from build123d import *

# Parameters (mm, degrees)
F1_DEPTH = 5
F3_D     = 5


with BuildPart() as f1:
    # F0 (on Top) → F1 (new body)
    with BuildSketch(Plane.XY):
        with BuildLine():
            Line((-14.706516, -4.991379), (-0.002931, -4.999999))
            ThreePointArc((-0.002931, -4.999999), (3.536527, -3.53454), (4.999997, 0.005741))
            Line((4.999997, 0.005741), (4.98325, 14.591081))
            Line((4.98325, 14.591081), (4.982298, 15.420361))
            ThreePointArc((4.982298, 15.420361), (-0.210367, 19.995573), (-5, 15))
            ThreePointArc((-5, 15), (-7.928932, 7.928932), (-15, 5))
            ThreePointArc((-15, 5), (-19.997844, -0.146805), (-14.706516, -4.991379))
        make_face()
        with BuildLine():
            Line((4.982298, 15.420361), (4.98325, 14.591081))
            ThreePointArc((4.98325, 14.591081), (4.999997, 15.005741), (4.982298, 15.420361))
        make_face()
    extrude(amount=F1_DEPTH)

    # F3 (through all)
    with Locations(Plane.XY.offset(5)):
        with Locations((0, 15), (-15, 0)):
            Hole(F3_D / 2)


solid = f1.part
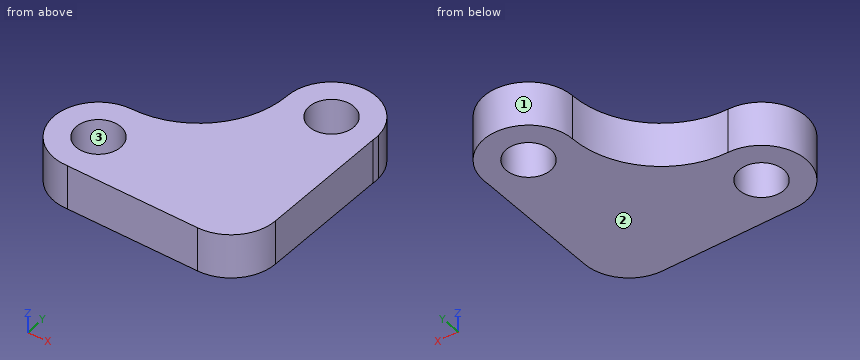
Model file for the job. Use its own axes, mm. Face numbers are marked on the shaded views. Give positions to 0.01 mm unless a question says otherwise; leave off trailing zeros. Loops run counter-clockwise (first coordinate to the right, second up) from the corner with the lowest first, then second, coordinate; pieces in that order, holes last.
1) Pull direction X, two halves, no side cores. Call the marked faces 1, 2 and 3: +X half, -X half, draft (parallel to the pull), parting line (faces both ways), or undercut.
2) Saw through at D-D (x = -11.5). Write the cut outline in (y, z).
3) Saw through at B-B (y = 16). Write the cut outline in (x, z).
4) Wall check: line 1 (Y direction, x = -15, z = 3); line 2 (Y direction, x = 0, z = 3.05); line 3 (Y direction, x = -8.25, z = 4.1). Give the ranges that are in metal, low to high.
5) Flat gauge pins, fed straight in: pin 1 Ø3 at (x, z) = (-10, 1) entering from -Y (3 decimals); pin 2 Ø3 at (x, y) = (-8.5, 14.5) entering from +Z. Where does each tip first touch, or does it go through?
6) Saw through at C-C (x = 1). Write the cut outline in (y, z).
7) Saw through at A-A (z = 1.9). Write the cut outline in (x, y).
Answer block:
1. face 1: parting line
1. face 2: draft
1. face 3: undercut
2. outline: (-4.99, 0) - (5.63, 0) - (5.63, 5) - (-4.99, 5) - close
3. outline: (-4.9, 0) - (-2.29, 0) - (-2.29, 5) - (-4.9, 5) - close; (2.29, 0) - (4.9, 0) - (4.9, 5) - (2.29, 5) - close
4. line 1: y = -5 to -2.5, 2.5 to 5
4. line 2: y = -5 to 12.5, 17.5 to 20
4. line 3: y = -5 to 7.62
5. pin 1: stops at y = -4.995
5. pin 2: passes through
6. outline: (-4.9, 0) - (12.71, 0) - (12.71, 5) - (-4.9, 5) - close; (17.29, 0) - (19.9, 0) - (19.9, 5) - (17.29, 5) - close
7. outline: (-15, 5) arc R5 ccw (long way) to (-14.71, -4.99) - (0, -5) arc R5 ccw to (5, 0.01) - (4.98, 14.59) arc R5 ccw to (4.98, 15.42) arc R5 ccw to (-5, 15) arc R10 cw to start; hole circle Ø5 at (-15, 0); hole circle Ø5 at (0, 15)
